The listing builds one solid part. Answer for the finished solid, in the listing's coordinates (mm). Face numbers are marked on the shaded views. A direction names the side the tool comes from. Round coordinates to 2 decimals unless told otherwise and drop trailing zeros. Order: outer loops, then holes, each group sorted by start corner. A loop starts at its lowest first (then second) coordinate and runs counter-clockwise, first axis right, second up. Notation, with made-up numbers: M 22,-8 L 75,-8 A24 cw 75,25 Z; hole C -3,83 d2. An arc over 180 degrees is marked long. Put each result on its own line as item: value. Start each with the question number.
1. The part is cut by section D-D (y = -68.5). Give the vertices of the cut face in (x, z), then the cut area to 3 significant figures.
2. The part is cut by section B-B (x = 167). Give the vertices of the cut face in (y, z), then the cut area to 3 significant figures.
3. The part is cut by section C-C (y = 370). Give the vertices of the cut face in (x, z), then the cut area to 3 significant figures.
4. Each of these flat-tipped pins is pushed along its axis until it touches: pin 1 Ø5 at (x, y) = (93, -27.5) entering from +Z; pin 2 Ø8 at (x, y) = (-92, 308) entering from +Z; pin 3 Ø10 at (x, y) = (191, -246) entering from -Z; pin 4 Ø6 at (y, z) = (-245, 211) entering from -X. Where does it stop, or does it pass through?
5. The mould has two halves that part along Z. Classify the marked faces 1, 2 and 3: +Z half, -Z half, draft (parallel to the pull), parting line (faces both ways), or undercut.
6. Which of the six approach directions +Z, -Z, +X, -X, +Y, -Y give full straight-line access (tool end or side, diameter ignored) to the marked faces 4, 5 and 6?
7. Consider line 1 (Y direction, x = -172, z = 90); line 2 (Y direction, x = -36, z = 205.5); line 3 (X direction, y = 383.5, z = 165). Determine where each line is inside the solid, lowest interval first.
8. The part is cut by section A-A (z = 165). Give the vertices of the cut face in (x, y), then the cut area to 3 significant figures.
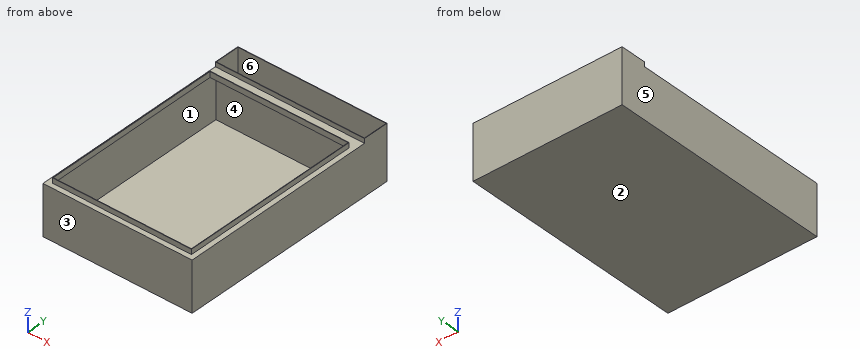
from build123d import *

# Parameters (mm, degrees)
SKETCH1_W           = 600
SKETCH1_H           = 900
BOSS_EXTRUDE1_DEPTH = 200
SHELL1_T            = -2
SKETCH2_W           = 596
SKETCH2_H           = 2
BOSS_EXTRUDE2_DEPTH = 198
SKETCH3_W           = 596
SKETCH3_H           = 794
SKETCH3_W_2         = 556
SKETCH3_H_2         = 724
BOSS_EXTRUDE3_DEPTH = 2
SKETCH4_W           = 560
SKETCH4_H           = 728
SKETCH4_W_2         = 556
SKETCH4_H_2         = 724
BOSS_EXTRUDE4_DEPTH = 20
SKETCH5_W           = 600
SKETCH5_H           = 104
SKETCH5_W_2         = 596
SKETCH5_H_2         = 100
BOSS_EXTRUDE5_DEPTH = 18


with BuildPart() as part:
    # Sketch1 → Boss-Extrude1 (new body)
    with BuildSketch(Plane.XY):
        Rectangle(SKETCH1_W, SKETCH1_H)
    extrude(amount=BOSS_EXTRUDE1_DEPTH)

    # Shell1
    shell1_openings = [part.faces().sort_by_distance(p)[0] for p in [
        (0, 0, 200),
    ]]
    offset(amount=SHELL1_T, openings=shell1_openings, kind=Kind.INTERSECTION)

    # Sketch2 → Boss-Extrude2 (add)
    with BuildSketch(Plane.XY.offset(2)):
        with Locations((0, 347)):
            Rectangle(SKETCH2_W, SKETCH2_H)
    extrude(amount=BOSS_EXTRUDE2_DEPTH)

    # Sketch3 → Boss-Extrude3 (add)
    with BuildSketch(Plane.XY.offset(200)):
        with Locations((0, -51)):
            Rectangle(SKETCH3_W, SKETCH3_H)
        with Locations((0, -66)):
            Rectangle(SKETCH3_W_2, SKETCH3_H_2, mode=Mode.SUBTRACT)
    extrude(amount=-BOSS_EXTRUDE3_DEPTH)

    # Sketch4 → Boss-Extrude4 (add)
    with BuildSketch(Plane.XY.offset(200)):
        with Locations((0, -66)):
            Rectangle(SKETCH4_W, SKETCH4_H)
        with Locations((0, -66)):
            Rectangle(SKETCH4_W_2, SKETCH4_H_2, mode=Mode.SUBTRACT)
    extrude(amount=BOSS_EXTRUDE4_DEPTH)

    # Sketch5 → Boss-Extrude5 (add)
    with BuildSketch(Plane.XY.offset(200)):
        with Locations((0, 398)):
            Rectangle(SKETCH5_W, SKETCH5_H)
        with Locations((0, 398)):
            Rectangle(SKETCH5_W_2, SKETCH5_H_2, mode=Mode.SUBTRACT)
    extrude(amount=BOSS_EXTRUDE5_DEPTH)


solid = part.part
Resolved:
1. outline: M -300,0 L 300,0 L 300,200 L 280,200 L 280,220 L 278,220 L 278,198 L 298,198 L 298,2 L -298,2 L -298,198 L -278,198 L -278,220 L -280,220 L -280,200 L -300,200 Z
1. area: 2,150 mm2
2. outline: M -450,0 L 450,0 L 450,218 L 448,218 L 448,2 L 348,2 L 348,218 L 346,218 L 346,200 L 298,200 L 298,220 L 296,220 L 296,198 L 346,198 L 346,2 L -448,2 L -448,198 L -428,198 L -428,220 L -430,220 L -430,200 L -450,200 Z
2. area: 3,280 mm2
3. outline: M -300,0 L 300,0 L 300,218 L 298,218 L 298,2 L -298,2 L -298,218 L -300,218 Z
3. area: 2,060 mm2
4. pin 1: z = 2
4. pin 2: z = 200
4. pin 3: z = 0
4. pin 4: x = -280
5. face 1: undercut
5. face 2: -Z half
5. face 3: draft
6. face 4: none
6. face 5: +Z, -Z, -X, +Y, -Y
6. face 6: +Z
7. line 1: -450 to -448, 346 to 348, 448 to 450
7. line 2: -430 to -428, 296 to 298, 346 to 348, 448 to 450
7. line 3: -300 to -298, 298 to 300
8. outline: M -300,-450 L 300,-450 L 300,450 L -300,450 Z; hole M -298,-448 L 298,-448 L 298,346 L -298,346 Z; hole M -298,348 L 298,348 L 298,448 L -298,448 Z
8. area: 7,180 mm2
